Source: CAD feature listing. Evaluate the final solid. Frame: model axes, mm. A direction names the side the tool comes from. Give positions to 0.01 mm unless a question says otherwise; leave off trailing zeros. Order: outer loops, then holes, each group sorted by start corner. A loop starts at its lowest first (then second) coordinate and runs counter-clockwise, first axis right, second up. Notation, with made-up numbers: M 56.5,37 L 111.5,37 A30 ccw 111.5,71 Z; hole C 86.25,67.25 d3. An arc over 180 degrees is marked long. Answer in a Markdown table with one row per item. Add a question column.
(1) Pin query (flat end, axial travel): P1, Ø1.5, axis at x = 16, y = -13.5, coming from the -Z side; P2, Ø10, axis at x = 12, y = 0.5, coming from the +Z side; P3, Ø7, axis at y = 27.5, z = 125.35, coming from the +X side. Return the tip coordinate at first contact, or that it passes through.
(2) Mould query, pull axis Y, two halves, no side actions, for faces 3 (the face through (5, 40.2, 28.9)), 4 (the face through (2, -1, -120.75)), 5 (the face through (12.395, -30.14, 1.719)). Classes: pulls with the +Y half, pulls with the -Y half, needs draft (parallel to the pull), parting line crosses it, or undercut.
(3) Section query A-A, the plane z = -125.35. Return loops of the section in (x, y).
(4) Section query D-D, the plane y = -33. Return loops of the section in (x, z).
(5) Section query C-C, the plane y = 6.5. Return loops of the section in (x, z), plus the area to 3 significant figures.
(6) Material intervals for line 1 along Y through (x, z) = (2.4, -125.35); line 2 along Y through (x, z) = (3.5, 90.5); line 3 along Z through (x, y) = (2.15, -27.5), sorted ascending.
(7) Section query B-B, the plane x = 13.25. Return loops of the section in (y, z).
(8) Set-up query: faces 1 (the face through (20, 19, 0)), 2 (the face through (2, -1, 120.75)). Return all of +Z, -Z, +X, -X, +Y, -Y with unobstructed straight access to the full face (end or side cutting, diameter ignored); none if empty.
from build123d import *

# Parameters (mm, degrees)
SKETCH1_W            = 255.1
SKETCH1_H            = 90
SKETCH1_W_2          = 241.5
SKETCH1_H_2          = 76
BOSS_EXTRUDE1_DEPTH  = 5
BOSS_EXTRUDE2_DEPTH  = 78
BOSS_EXTRUDE3_DEPTH  = 2
BOSS_EXTRUDE4_DEPTH  = 241.5
CUT_EXTRUDE1_DEPTH   = 141
CUT_EXTRUDE2_DEPTH   = 141
M4_CLEARANCE_HOLE1_D = 4.5


with BuildPart() as part:
    # Sketch1 → Boss-Extrude1 (new body)
    with BuildSketch(Plane(origin=(0, 0, 0), x_dir=(0, 0, -1), z_dir=(1, 0, 0))):
        Rectangle(SKETCH1_W, SKETCH1_H)
        Rectangle(SKETCH1_W_2, SKETCH1_H_2, mode=Mode.SUBTRACT)
    extrude(amount=BOSS_EXTRUDE1_DEPTH)

    # Sketch3 → Boss-Extrude2 (add)
    with BuildSketch(Plane(origin=(0, -38, 0), x_dir=(1, 0, 0), z_dir=(0, 1, 0))):
        Polygon((5, 120.75), (20, 83.75), (20, 85.75), (5, 122.75), align=None)
    boss_extrude2 = extrude(amount=BOSS_EXTRUDE2_DEPTH)

    # Sketch6 → Boss-Extrude3 (add)
    with BuildSketch(Plane.XZ.offset(38)):
        Polygon((5, -122.75), (20, -85.75), (20, -83.75), (5, -120.75), align=None)
    boss_extrude3 = extrude(amount=BOSS_EXTRUDE3_DEPTH)

    # Mirror1: Boss-Extrude2, Boss-Extrude3 across plane
    add(boss_extrude2.mirror(Plane.XY))
    add(boss_extrude3.mirror(Plane.XY))

    # Sketch7 → Boss-Extrude4 (add)
    with BuildSketch(Plane.XY.offset(-120.75)):
        Polygon((5, 38), (20, 18), (20, 20), (5, 40), align=None)
        Polygon((5, -40), (5, -38), (20, -18), (20, -20), align=None)
    extrude(amount=BOSS_EXTRUDE4_DEPTH)

    # Sketch8 → Cut-Extrude1 (cut)
    with BuildSketch(Plane.XZ.offset(45)):
        Polygon((20, -120.75), (5.810810811, -120.75), (20, -85.75), align=None)
        Polygon((5.810810811, 120.75), (20, 120.75), (20, 85.75), align=None)
    extrude(amount=-CUT_EXTRUDE1_DEPTH, mode=Mode.SUBTRACT)

    # Sketch9 → Cut-Extrude2 (cut, symmetric)
    with BuildSketch(Plane.XY):
        Polygon((5, 40), (20, 20), (20, 40), align=None)
    cut_extrude2 = extrude(amount=CUT_EXTRUDE2_DEPTH, both=True, mode=Mode.SUBTRACT)

    # Mirror5: Cut-Extrude2 across plane
    add(cut_extrude2.mirror(Plane.ZX), mode=Mode.SUBTRACT)

    # M4 Clearance Hole1 (through all)
    with Locations(Plane(origin=(5, 0, 0), x_dir=(0, 0, -1), z_dir=(1, 0, 0))):
        with Locations((-125.35, 27.5), (-125.35, -27.5)):
            m4_clearance_hole1 = Hole(M4_CLEARANCE_HOLE1_D / 2)

    # Mirror6: M4 Clearance Hole1 across plane
    add(m4_clearance_hole1.mirror(Plane.XY), mode=Mode.SUBTRACT)


solid = part.part
Values follow:
| question | item | result |
|---|---|---|
| 1 | P1 | stops at z = -97.47 |
| 1 | P2 | stops at z = 117.82 |
| 1 | P3 | stops at x = 5.36 |
| 2 | face 3 | needs draft |
| 2 | face 4 | undercut |
| 2 | face 5 | pulls with the -Y half |
| 3 | outline | M 0,-45 L 5,-45 L 5,-29.75 L 0,-29.75 Z; M 0,-25.25 L 5,-25.25 L 5,25.25 L 0,25.25 Z; M 0,29.75 L 5,29.75 L 5,45 L 0,45 Z |
| 4 | outline | M 0,-127.55 L 5,-127.55 L 5,-122.75 L 10.25,-109.8 L 10.25,109.8 L 5,122.75 L 5,127.55 L 0,127.55 L 0,120.75 L 5,120.75 L 8.75,111.5 L 8.75,-111.5 L 5,-120.75 L 0,-120.75 Z |
| 5 | outline | M 0,-127.55 L 5,-127.55 L 5,-122.75 L 20,-85.75 L 20,-83.75 L 5,-120.75 L 0,-120.75 Z; M 0,120.75 L 5,120.75 L 20,83.75 L 20,85.75 L 5,122.75 L 5,127.55 L 0,127.55 Z |
| 5 | area | 128 mm² |
| 6 | line 1 | y = -45 to -29.75, -25.25 to 25.25, 29.75 to 45 |
| 6 | line 2 | y = -45 to -38, 38 to 45 |
| 6 | line 3 | z = -123.1 to -120.75, 120.75 to 123.1 |
| 7 | outline | M -29,-102.4 L 29,-102.4 L 29,102.4 L -29,102.4 Z; hole M -27,-100.4 L 27,-100.4 L 27,100.4 L -27,100.4 Z |
| 8 | face 1 | +Z, -Z, +X, +Y, -Y |
| 8 | face 2 | -X |
